from build123d import *

# Parameters (mm, degrees)
F0_W      = 47
F0_H      = 31
F1_DEPTH  = 15
F2_R      = 1.9
F3_DEPTH  = 60
F5_DEPTH  = 70
F6_R      = 1.9
F7_DEPTH  = 80
F9_DEPTH  = 70
F11_DEPTH = 70


with BuildPart() as f1:
    # F0 (on Front) → F1 (new body)
    with BuildSketch(Plane.XZ):
        with Locations((-69.120786, -3.705296)):
            Rectangle(F0_W, F0_H)
    extrude(amount=F1_DEPTH)

    # F2 (on face) → F3 (cut)
    with BuildSketch(Plane(origin=(0, 0, -19.205296), x_dir=(1, 0, 0), z_dir=(0, 0, -1))):
        with Locations((-51.120786, 7.5)):
            Circle(F2_R)
    extrude(amount=-F3_DEPTH, mode=Mode.SUBTRACT)

    # F4 (on face) → F5 (cut)
    with BuildSketch(Plane(origin=(0, 0, -19.205296), x_dir=(1, 0, 0), z_dir=(0, 0, -1))):
        with BuildLine():
            ThreePointArc((-84.706673, 0), (-92.206673, 7.5), (-84.706673, 15))
            Line((-84.706673, 15), (-92.620786, 15))
            Line((-92.620786, 15), (-92.620786, 0))
            Line((-92.620786, 0), (-84.706673, 0))
        make_face()
    extrude(amount=-F5_DEPTH, mode=Mode.SUBTRACT)

    # F6 (on face) → F7 (cut)
    with BuildSketch(Plane(origin=(0, 0, -19.205296), x_dir=(1, 0, 0), z_dir=(0, 0, -1))):
        with Locations((-86.707558, 7.5987)):
            Circle(F6_R)
    extrude(amount=-F7_DEPTH, mode=Mode.SUBTRACT)

    # F8 (on face) → F9 (cut)
    with BuildSketch(Plane(origin=(0, 0, -19.205296), x_dir=(1, 0, 0), z_dir=(0, 0, -1))):
        with BuildLine():
            Line((-45.620786, 0), (19.677406, 0))
            ThreePointArc((19.677406, 0), (27.177406, 7.5), (19.677406, 15))
            Line((19.677406, 15), (-45.620786, 15))
            Line((-45.620786, 15), (-45.620786, 0))
        make_face()
    extrude(amount=-F9_DEPTH, mode=Mode.SUBTRACT)

    # F10 (on face) → F11 (cut)
    with BuildSketch(Plane.XY.offset(11.794704)):
        with BuildLine():
            ThreePointArc((-53.020786, 0), (-48.168205, -1.781394), (-45.620786, -6.279344))
            Line((-45.620786, -6.279344), (-45.620786, 0))
            Line((-45.620786, 0), (-53.020786, 0))
        make_face()
        with BuildLine():
            Line((-45.620786, -6.279344), (-45.620786, -8.720656))
            ThreePointArc((-45.620786, -8.720656), (-45.520786, -7.5), (-45.620786, -6.279344))
        make_face()
        with BuildLine():
            ThreePointArc((-45.620786, -8.720656), (-48.168205, -13.218606), (-53.020786, -15))
            Line((-53.020786, -15), (-45.620786, -15))
            Line((-45.620786, -15), (-45.620786, -8.720656))
        make_face()
    extrude(amount=-F11_DEPTH, mode=Mode.SUBTRACT)


solid = f1.part
Geometry check sheet. Reference: the model listing, model coordinates, mm. Give positions to 0.01 mm unless a question says otherwise; leave off trailing zeros. Loops run counter-clockwise (first coordinate to the right, second up) from the corner with the lowest first, then second, coordinate; pieces in that order, holes last. Notation, with made-up numbers: M -7,25 L 10,25 A15 cw 10,43 Z; hole C 3,65.5 d7. An arc over 180 degrees is marked long. Answer as a JSON object with one key per item and string values. Group by question number.
Item 1: Mould release check, pull along Y, two halves, no side actions. Record for faces 1 (the cylindrical face through (-49.366, -6.772, -3.922)), 2 (the flat face through (-45.621, -7, -4)), 3 (the cylindrical face through (-92.205, -7.335, -3.922)): pulls with the +Y half, pulls with the -Y half, needs draft (parallel to the pull), parting line crosses it, or undercut.
Item 2: Material ranges on L1, parallel to X at y = -7.5, z = -7.5 (3 decimals); L2, parallel to X at y = -8.75, z = 8; L3, parallel to Y at x = -88, z = 7.5, recorded low to high.
Item 3: Sectioned sample at B-B on z = 8. Record the boundary of the cut face in (x, y), plus the area to 3 significant figures.
Item 4: Gauge pin test, flat ends, axial feed: pin 1 (4 mm diameter, centred on y = -4, z = -12, fed in from -X); pin 2 (5 mm diameter, centred on y = -10.5, z = -14, fed in from -X). Record the tip position at first contact, or that the pin passes through.
Item 5: Sectioned sample at C-C on x = -86. Record the boundary of the cut face in (y, z), plus the area to 3 significant figures.
Item 6: Sectioned sample at D-D on y = -13.25. Record the boundary of the cut face in (x, z).
Item 7: Sectioned sample at A-A on x = -51. Record the boundary of the cut face in (y, z), plus the area to 3 significant figures.
Findings below:
{
 "1": {"face 1": "undercut", "face 2": "needs draft", "face 3": "parting line crosses it"},
 "2": {"L1": "-92.207 to -88.605, -84.81 to -53.021, -49.221 to -45.621", "L2": "-92.1 to -88.22, -85.2 to -52.55, -49.69 to -45.63", "L3": "-14.24 to -8.99, -6.21 to -0.76"},
 "3": {"outline": "M -84.71,-15 L -53.02,-15 A7.5 ccw -45.62,-8.72 L -45.62,-6.28 A7.5 ccw -53.02,0 L -84.71,0 A7.5 ccw Z; hole C -86.71,-7.6 d3.8; hole C -51.12,-7.5 d3.8", "area": "629 mm2"},
 "4": {"pin 1": "x = -92.06", "pin 2": "x = -92.19"},
 "5": {"outline": "M -14.89,-19.21 L -9.36,-19.21 L -9.36,11.79 L -14.89,11.79 Z; M -5.84,-19.21 L -0.11,-19.21 L -0.11,11.79 L -5.84,11.79 Z", "area": "349 mm2"},
 "6": {"outline": "M -89.52,-19.21 L -48.21,-19.21 L -48.21,11.79 L -89.52,11.79 Z"},
 "7": {"outline": "M -14.72,-19.21 L -9.4,-19.21 L -9.4,11.79 L -14.72,11.79 Z; M -5.6,-19.21 L -0.28,-19.21 L -0.28,11.79 L -5.6,11.79 Z", "area": "330 mm2"}
}
